from build123d import *

# Parameters (mm, degrees)
SKETCH_1_W          = 15.4
SKETCH_1_H          = 15.4
EXTRUDE_1_DEPTH     = 3
SKETCH_3_R          = 1.6
CUT_EXTRUDE_1_DEPTH = 31.413812651


with BuildPart() as part:
    # 草图1 → 凸台-拉伸1 (new, symmetric)
    with BuildSketch(Plane(origin=(0, 0, 0), x_dir=(0, 0, -1), z_dir=(1, 0, 0))):
        with BuildLine():
            Line((13.416407865, 4), (13.416407865, -4))
            ThreePointArc((13.416407865, -4), (0, -14), (-13.416407865, -4))
            Line((-13.416407865, -4), (-13.416407865, 4))
            ThreePointArc((-13.416407865, 4), (0, 14), (13.416407865, 4))
        make_face()
        Rectangle(SKETCH_1_W, SKETCH_1_H, mode=Mode.SUBTRACT)
    extrude(amount=EXTRUDE_1_DEPTH, both=True)

    # 草图3 → 切除-拉伸1 (cut, through all)
    with BuildSketch(Plane.XY.offset(13.416407865)):
        Circle(SKETCH_3_R)
    extrude(amount=-CUT_EXTRUDE_1_DEPTH, mode=Mode.SUBTRACT)


solid = part.part
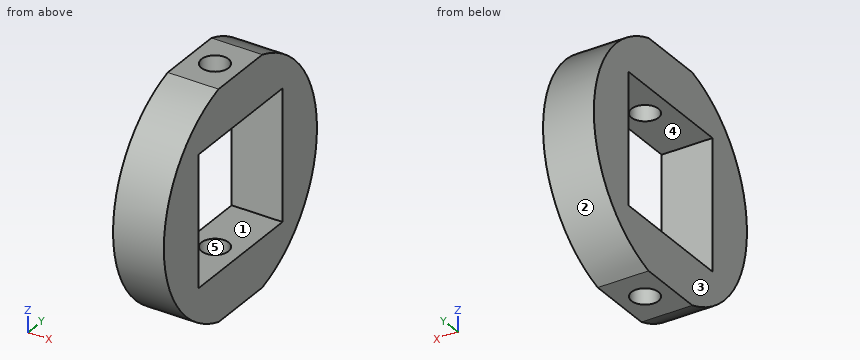
The model under review builds one solid part; all positions refer to its coordinate system, in mm. Face numbers are marked on the shaded views. A direction names the side the tool comes from. Round coordinates to 2 decimals unless told otherwise and drop trailing zeros. Loops run counter-clockwise (first coordinate to the right, second up) from the corner with the lowest first, then second, coordinate; pieces in that order, holes last. Notation, with made-up numbers: (-33, -11.75) -> (-13, -11.75) arc R10 cw to (-13, 2.25) -> close; hole circle Ø11 at (-11, -0.5). An arc over 180 degrees is marked (long way). Write item = value, one per line. Start each with the question number.
Item 1: Take a section at A-A on y = 0. Give the boundary of the cut face in (x, z), plus the area to 3 significant figures.
Item 2: Take a section at B-B on x = -0.95. Give the boundary of the cut face in (y, z), plus the area to 3 significant figures.
Item 3: Take a section at D-D on z = -1.25. Give the boundary of the cut face in (x, y).
Item 4: For the marked faces 1 and 2, list the 3-axis set-ups (+Z, -Z, +X, -X, +Y, -Y) from which the entire face can be reached by the end or side of a thin tool; tool diameter is ignored.
Item 5: Insertion check: pin 1 (1 mm diameter, centred on x = 0, y = 5.5, fed in from -Z); pin 2 (1.5 mm diameter, centred on x = -2, z = 6, fed in from -Y); pin 3 (1 mm diameter, centred on x = 0, y = -6.5, fed in from -Z). Each pin has a flat end and moves straight along its axis. Give the tip position at first contact, or say it passes through.
Item 6: Take a section at C-C on y = -6.75. Give the boundary of the cut face in (x, z).
Item 7: Mouldability with a two-part tool opening along X and no side actions: class the marked faces 3, 4 and 5 as released by +X, released by -X, zero draft, split by the parting line, or undercut.
Item 8: To check wall thickness, follow L1, parallel to Y at x = 2.3, z = 4; L2, parallel to Y at x = -1.9, z = -7.25. State the ranges of each line that lie inside material, in increasing order.
Result:
q1.outline = (-3, -13.42) -> (-1.6, -13.42) -> (-1.6, -7.7) -> (-3, -7.7) -> close; (-3, 7.7) -> (-1.6, 7.7) -> (-1.6, 13.42) -> (-3, 13.42) -> close; (1.6, -13.42) -> (3, -13.42) -> (3, -7.7) -> (1.6, -7.7) -> close; (1.6, 7.7) -> (3, 7.7) -> (3, 13.42) -> (1.6, 13.42) -> close
q1.area = 32.0 mm²
q2.outline = (-7.7, -7.7) -> (-7.7, 7.7) -> (-1.29, 7.7) -> (-1.29, 13.42) -> (-4, 13.42) arc R14 ccw to (-4, -13.42) -> (-1.29, -13.42) -> (-1.29, -7.7) -> close; (1.29, -13.42) -> (4, -13.42) arc R14 ccw to (4, 13.42) -> (1.29, 13.42) -> (1.29, 7.7) -> (7.7, 7.7) -> (7.7, -7.7) -> (1.29, -7.7) -> close
q2.area = 343 mm²
q3.outline = (-3, -13.94) -> (3, -13.94) -> (3, -7.7) -> (-3, -7.7) -> close; (-3, 7.7) -> (3, 7.7) -> (3, 13.94) -> (-3, 13.94) -> close
q4.face_1 = +X, -X
q4.face_2 = +X, -X, +Y
q5.pin_1 = -13.08
q5.pin_2 = -12.98
q5.pin_3 = -12.65
q6.outline = (-3, -12.27) -> (3, -12.27) -> (3, -7.7) -> (-3, -7.7) -> close; (-3, 7.7) -> (3, 7.7) -> (3, 12.27) -> (-3, 12.27) -> close
q7.face_3 = released by -X
q7.face_4 = zero draft
q7.face_5 = undercut
q8.L1 = -13.42 to -7.7, 7.7 to 13.42
q8.L2 = -11.98 to -7.7, 7.7 to 11.98
